from build123d import *

# Parameters (mm, degrees)
SKETCH1_R                       = 15.113
BOSS_EXTRUDE1_DEPTH             = 6.35
FILLET1_R                       = 76.2
F_1_4_0_25_DIAMETER_SLOT1_DEPTH = 6.35
SKETCH4_R                       = 3.3655
CUT_EXTRUDE1_DEPTH              = 885.657788357
CIRPATTERN1_COUNT               = 4
CIRPATTERN1_ANGLE               = 60.5
CIRPATTERN1_THE_OTHER_WAY_COUNT = 4
CIRPATTERN1_THE_OTHER_WAY_ANGLE = 60.5
CUT_EXTRUDE2_DEPTH              = 885.657788357


# Read off the part's stored shape, not the designer's step: 1/4 (0.25) Diameter Slot1
with BuildPart() as part:
    # Sketch1 → Boss-Extrude1 (new body)
    with BuildSketch(Plane(origin=(0, 0, 0), x_dir=(0, 0, -1), z_dir=(1, 0, 0))):
        with BuildLine():
            Line((-558.8, 304.8), (-558.8, 685.8))
            Line((-558.8, 685.8), (558.8, 685.8))
            Line((558.8, 685.8), (558.8, 304.8))
            ThreePointArc((558.8, 304.8), (492.779998657, 124.430002015), (325.91999876, 29.300000517))
            Line((325.91999876, 29.300000517), (152.4, 0))
            Line((152.4, 0), (-152.4, 0))
            Line((-152.4, 0), (-325.91999876, 29.300000517))
            ThreePointArc((-325.91999876, 29.300000517), (-492.779998657, 124.430002015), (-558.8, 304.8))
        make_face()
        with Locations((-508, 342.9)):
            Circle(SKETCH1_R, mode=Mode.SUBTRACT)
        with Locations((508, 342.9)):
            Circle(SKETCH1_R, mode=Mode.SUBTRACT)
    extrude(amount=BOSS_EXTRUDE1_DEPTH)

    # Fillet1
    fillet1_edges = [part.edges().sort_by_distance(p)[0] for p in [
        (3.175, 685.8, 558.8),
        (3.175, 685.8, -558.8),
    ]]
    fillet(fillet1_edges, radius=FILLET1_R)

    # 1/4 (0.25) Diameter Slot1 outline → 1/4 (0.25) Diameter Slot1 (cut)
    with BuildSketch(Plane.YZ):
        with BuildLine():
            Line((47.625, -177.8), (34.925, -177.8))
            ThreePointArc((34.925, -177.8), (31.75, -180.975), (34.925, -184.15))
            Line((34.925, -184.15), (47.625, -184.15))
            ThreePointArc((47.625, -184.15), (50.8, -180.975), (47.625, -177.8))
        make_face()
        with BuildLine():
            ThreePointArc((164.719, -177.8), (161.544, -180.975), (164.719, -184.15))
            Line((164.719, -184.15), (177.419, -184.15))
            ThreePointArc((177.419, -184.15), (180.594, -180.975), (177.419, -177.8))
            Line((177.419, -177.8), (164.719, -177.8))
        make_face()
        with BuildLine():
            Line((47.625, -133.35), (34.925, -133.35))
            ThreePointArc((34.925, -133.35), (31.75, -136.525), (34.925, -139.7))
            Line((34.925, -139.7), (47.625, -139.7))
            ThreePointArc((47.625, -139.7), (50.8, -136.525), (47.625, -133.35))
        make_face()
        with BuildLine():
            ThreePointArc((164.719, -133.35), (161.544, -136.525), (164.719, -139.7))
            Line((164.719, -139.7), (177.419, -139.7))
            ThreePointArc((177.419, -139.7), (180.594, -136.525), (177.419, -133.35))
            Line((177.419, -133.35), (164.719, -133.35))
        make_face()
        with BuildLine():
            Line((177.419, 139.7), (164.719, 139.7))
            ThreePointArc((164.719, 139.7), (161.544, 136.525), (164.719, 133.35))
            Line((164.719, 133.35), (177.419, 133.35))
            ThreePointArc((177.419, 133.35), (180.594, 136.525), (177.419, 139.7))
        make_face()
        with BuildLine():
            ThreePointArc((34.925, 139.7), (31.75, 136.525), (34.925, 133.35))
            Line((34.925, 133.35), (47.625, 133.35))
            ThreePointArc((47.625, 133.35), (50.8, 136.525), (47.625, 139.7))
            Line((47.625, 139.7), (34.925, 139.7))
        make_face()
        with BuildLine():
            Line((47.625, 184.15), (34.925, 184.15))
            ThreePointArc((34.925, 184.15), (31.75, 180.975), (34.925, 177.8))
            Line((34.925, 177.8), (47.625, 177.8))
            ThreePointArc((47.625, 177.8), (50.8, 180.975), (47.625, 184.15))
        make_face()
        with BuildLine():
            ThreePointArc((164.719, 184.15), (161.544, 180.975), (164.719, 177.8))
            Line((164.719, 177.8), (177.419, 177.8))
            ThreePointArc((177.419, 177.8), (180.594, 180.975), (177.419, 184.15))
            Line((177.419, 184.15), (164.719, 184.15))
        make_face()
    extrude(amount=F_1_4_0_25_DIAMETER_SLOT1_DEPTH, mode=Mode.SUBTRACT)

    # Sketch4 → Cut-Extrude1 (cut, through all)
    with BuildSketch(Plane(origin=(6.35, 0, 0), x_dir=(0, 0, -1), z_dir=(1, 0, 0))):
        with Locations((0, 41.154707227)):
            Circle(SKETCH4_R)
        with Locations((0, 25.279707227)):
            Circle(SKETCH4_R)
    cut_extrude1 = extrude(amount=-CUT_EXTRUDE1_DEPTH, mode=Mode.SUBTRACT)

    # CirPattern1: Cut-Extrude1 ×4 about axis
    cirpattern1_axis = Axis((0, 604.717207227, 0), (-1, 0, 0))
    for i in range(1, CIRPATTERN1_COUNT):
        add(cut_extrude1.rotate(cirpattern1_axis, i * CIRPATTERN1_ANGLE / (CIRPATTERN1_COUNT - 1)), mode=Mode.SUBTRACT)

    # CirPattern1 the other way: Cut-Extrude1 ×4 about axis
    cirpattern1_the_other_way_axis = Axis((0, 604.717207227, 0), (1, 0, 0))
    for i in range(1, CIRPATTERN1_THE_OTHER_WAY_COUNT):
        add(cut_extrude1.rotate(cirpattern1_the_other_way_axis, i * CIRPATTERN1_THE_OTHER_WAY_ANGLE / (CIRPATTERN1_THE_OTHER_WAY_COUNT - 1)), mode=Mode.SUBTRACT)

    # Sketch6 → Cut-Extrude2 (cut, through all)
    with BuildSketch(Plane(origin=(6.35, 0, 0), x_dir=(0, 0, -1), z_dir=(1, 0, 0))):
        with BuildLine():
            Line((-25.4, 107.95), (25.4, 107.95))
            ThreePointArc((25.4, 107.95), (50.8, 82.55), (25.4, 57.15))
            Line((25.4, 57.15), (-25.4, 57.15))
            ThreePointArc((-25.4, 57.15), (-50.8, 82.55), (-25.4, 107.95))
        make_face()
    extrude(amount=-CUT_EXTRUDE2_DEPTH, mode=Mode.SUBTRACT)


solid = part.part
Read the model definition and answer for the solid it produces. Units are mm, in the model's axes. A direction names the side the tool comes from. Give positions to 0.01 mm unless a question says otherwise; leave off trailing zeros. Write each loop counter-clockwise with the first axis right and the second up, starting at its lowest first coordinate (ties: lowest second). Pieces come first, ordered by that corner, then holes. Notation, with made-up numbers: (80, 75) - (135, 75) arc R11 ccw to (135, 83) - close; hole circle Ø7 at (59.25, -39.5). An arc over 180 degrees is marked (long way). Return JSON: item names as keys, results as strings.
Q1. Consider line 1 along Y through (x, z) = (4.25, -24); line 2 along Y through (x, z) = (2.25, -34.5); line 3 along Y through (x, z) = (2.5, 283.5). Determine where each line is inside the solid, lowest interval first. Write a range as [from, to].
Reply:
{"line 1": "[0, 57.15], [107.95, 685.8]", "line 2": "[0, 58.84], [106.26, 685.8]", "line 3": "[22.14, 685.8]"}
Q2. A cutting plane is placed at D-D, the plane y = 644.5. Determine the outline of the cut face in (x, z), and give its area (3 significant figures).
Reply:
{"outline": "(0, -550.34) - (6.35, -550.34) - (6.35, 550.34) - (0, 550.34) - close", "area": "6,990 mm²"}
Q3. A cutting plane is placed at C-C, the plane z = 220. Determine the outline of the cut face in (x, y).
Reply:
{"outline": "(0, 11.41) - (6.35, 11.41) - (6.35, 685.8) - (0, 685.8) - close"}
Q4. A cutting plane is placed at B-B, the plane x = 5.25. Count the separate pieces of the cut face and the enclosed holes in it, and give its area (3 significant figures).
Reply:
{"separate pieces": "1", "enclosed holes": "25", "area": "706,000 mm²"}
Q5. For faces 1 (the face through (3.219, 83.109, -50.794)), 2 (the face through (3.131, 14.855, -240.375)), determine the directions among +Z, -Z, +X, -X, +Y, -Y from which every point of the face is accessible in a straight line to the end or side of a thin tool.
Reply:
{"face 1": "+X, -X", "face 2": "-Z, +X, -X, -Y"}
Q6. A cutting plane is placed at A-A, the plane y = 342.9. Determine the outline of the cut face in (x, z).
Reply:
{"outline": "(0, -558.8) - (6.35, -558.8) - (6.35, -523.11) - (0, -523.11) - close; (0, -492.89) - (6.35, -492.89) - (6.35, 492.89) - (0, 492.89) - close; (0, 523.11) - (6.35, 523.11) - (6.35, 558.8) - (0, 558.8) - close"}
Q7. For a pull along Z with two mould halves and no side action, classify faces 3 (the face through (3.131, 126.535, -494.542)), 4 (the face through (6.35, 348, -8)), 5 (the face through (3.219, 81.991, 50.794)) as released by +Z, released by -Z, zero draft, split by the parting line, or undercut.
Reply:
{"face 3": "released by -Z", "face 4": "zero draft", "face 5": "undercut"}
Q8. Given P1, Ø3, axis at x = 4, y = 274.5, coming from the -Z side; P2, Ø6, axis at y = 60.8, z = -199.76, coming from the +X side; P3, Ø3, axis at x = 4.5, y = 170.5, coming from the +Z side; P4, Ø3, axis at x = 4.5, y = 173.5, coming from the +Z side, each flat-ended and moving along its own axis, determine where each tip first touches the part or whether it passes through.
Reply:
{"P1": "z = -557.31", "P2": "through", "P3": "z = 525.22", "P4": "z = 526.82"}
